from build123d import *

# Parameters (mm, degrees)
SKETCH1_R               = 60
BOSS_EXTRUDE1_DEPTH     = 1.5
SKETCH2_R               = 1.6
CUT_EXTRUDE1_DEPTH      = 2.5
MIRROR2_COPY_1_SKETCH_R = 1.6
MIRROR2_COPY_1_DEPTH    = 2.5
SKETCH3_W               = 3
SKETCH3_H               = 4
CUT_EXTRUDE2_DEPTH      = 4
LPATTERN1_COUNT         = 2
LPATTERN1_PITCH         = 8
MIRROR3_COPY_1_SKETCH_W = 3
MIRROR3_COPY_1_SKETCH_H = 4
MIRROR3_COPY_1_DEPTH    = 4
MIRROR4_COPY_1_SKETCH_W = 3
MIRROR4_COPY_1_SKETCH_H = 4
MIRROR4_COPY_1_DEPTH    = 4
MIRROR4_COPY_2_SKETCH_W = 3
MIRROR4_COPY_2_SKETCH_H = 4
MIRROR4_COPY_2_DEPTH    = 4
MIRROR4_COPY_3_SKETCH_W = 3
MIRROR4_COPY_3_SKETCH_H = 4
MIRROR4_COPY_3_DEPTH    = 4
CUT_EXTRUDE3_START      = -4
CUT_EXTRUDE3_DEPTH      = 5
CIRPATTERN1_COUNT       = 4


with BuildPart() as part:
    # Sketch1 → Boss-Extrude1 (new body, symmetric)
    with BuildSketch(Plane(origin=(0, 0, 0), x_dir=(1, 0, 0), z_dir=(0, 1, 0))):
        Circle(SKETCH1_R)
    extrude(amount=BOSS_EXTRUDE1_DEPTH, both=True)

    # Sketch2 → Cut-Extrude1 (cut, symmetric)
    with BuildSketch(Plane(origin=(0, 0, 0), x_dir=(1, 0, 0), z_dir=(0, 1, 0))):
        with Locations((54, 11)):
            Circle(SKETCH2_R)
    cut_extrude1 = extrude(amount=CUT_EXTRUDE1_DEPTH, both=True, mode=Mode.SUBTRACT)

    # Mirror1: Cut-Extrude1 across plane
    add(cut_extrude1.mirror(Plane(origin=(0, 0, 0), x_dir=(0, 0, 1), z_dir=(1, 0, 0))), mode=Mode.SUBTRACT)

    # Mirror2: Cut-Extrude1 across plane
    add(cut_extrude1.mirror(Plane.XY), mode=Mode.SUBTRACT)

    # Mirror2 copy 1 sketch → Mirror2 copy 1 (cut, symmetric)
    with BuildSketch(Plane(origin=(0, 0, 0), x_dir=(-1, 0, 0), z_dir=(0, 1, 0))):
        with Locations((54, 11)):
            Circle(MIRROR2_COPY_1_SKETCH_R)
    extrude(amount=MIRROR2_COPY_1_DEPTH, both=True, mode=Mode.SUBTRACT)

    # Sketch3 → Cut-Extrude2 (cut, through all)
    with BuildSketch(Plane(origin=(0, 1.5, 0), x_dir=(1, 0, 0), z_dir=(0, 1, 0))):
        with Locations((-8.5, 48)):
            Rectangle(SKETCH3_W, SKETCH3_H)
    cut_extrude2 = extrude(amount=-CUT_EXTRUDE2_DEPTH, mode=Mode.SUBTRACT)

    # LPattern1: Cut-Extrude2 ×2
    with Locations(*[(0, 0, i * LPATTERN1_PITCH) for i in range(1, LPATTERN1_COUNT)]):
        add(cut_extrude2, mode=Mode.SUBTRACT)

    # Mirror3: Cut-Extrude2 across plane
    add(cut_extrude2.mirror(Plane(origin=(0, 0, 0), x_dir=(0, 0, 1), z_dir=(1, 0, 0))), mode=Mode.SUBTRACT)

    # Mirror3 copy 1 sketch → Mirror3 copy 1 (cut, through all)
    with BuildSketch(Plane(origin=(0, 1.5, 8), x_dir=(-1, 0, 0), z_dir=(0, 1, 0))):
        with Locations((-8.5, -48)):
            Rectangle(MIRROR3_COPY_1_SKETCH_W, MIRROR3_COPY_1_SKETCH_H)
    extrude(amount=-MIRROR3_COPY_1_DEPTH, mode=Mode.SUBTRACT)

    # Mirror4: Cut-Extrude2 across plane
    add(cut_extrude2.mirror(Plane.XY), mode=Mode.SUBTRACT)

    # Mirror4 copy 1 sketch → Mirror4 copy 1 (cut, through all)
    with BuildSketch(Plane(origin=(0, 1.5, 0), x_dir=(-1, 0, 0), z_dir=(0, 1, 0))):
        with Locations((-8.5, 48)):
            Rectangle(MIRROR4_COPY_1_SKETCH_W, MIRROR4_COPY_1_SKETCH_H)
    extrude(amount=-MIRROR4_COPY_1_DEPTH, mode=Mode.SUBTRACT)

    # Mirror4 copy 2 sketch → Mirror4 copy 2 (cut, through all)
    with BuildSketch(Plane(origin=(0, 1.5, -8), x_dir=(-1, 0, 0), z_dir=(0, 1, 0))):
        with Locations((-8.5, 48)):
            Rectangle(MIRROR4_COPY_2_SKETCH_W, MIRROR4_COPY_2_SKETCH_H)
    extrude(amount=-MIRROR4_COPY_2_DEPTH, mode=Mode.SUBTRACT)

    # Mirror4 copy 3 sketch → Mirror4 copy 3 (cut, through all)
    with BuildSketch(Plane(origin=(0, 1.5, -8), x_dir=(1, 0, 0), z_dir=(0, 1, 0))):
        with Locations((-8.5, -48)):
            Rectangle(MIRROR4_COPY_3_SKETCH_W, MIRROR4_COPY_3_SKETCH_H)
    extrude(amount=-MIRROR4_COPY_3_DEPTH, mode=Mode.SUBTRACT)

    # Sketch4 → Cut-Extrude3 (cut)
    with BuildSketch(Plane(origin=(0, 1.5, 0), x_dir=(1, 0, 0), z_dir=(0, 1, 0)).offset(CUT_EXTRUDE3_START)):
        Polygon((27.223611076, 41.365746699), (41.365746699, 27.223611076), (43.487067043, 29.344931419), (29.344931419, 43.487067043), align=None)
    cut_extrude3 = extrude(amount=CUT_EXTRUDE3_DEPTH, mode=Mode.SUBTRACT)

    # CirPattern1: Cut-Extrude3 ×4 about axis
    cirpattern1_axis = Axis((0, 0, 0), (0, 1, 0))
    for i in range(1, CIRPATTERN1_COUNT):
        add(cut_extrude3.rotate(cirpattern1_axis, i * 360 / CIRPATTERN1_COUNT), mode=Mode.SUBTRACT)


solid = part.part
For this review, take the finished solid that the model builds, in its own axes (mm). Coordinates: 2 decimals unless noted, no trailing zeros. Loops run counter-clockwise (first coordinate to the right, second up) from the corner with the lowest first, then second, coordinate; pieces in that order, holes last. Notation, with made-up numbers: (15, 82) - (20, 82) arc R34 cw to (20, 121) - close; hole circle Ø3 at (34.5, -37). An arc over 180 degrees is marked (long way). Use a Markdown table: item, result. Add a question column.
Item 1: For line 1 (Z direction, x = 54, y = -0.7); line 2 (X direction, y = -0.3, z = -43); line 3 (Z direction, x = -36.5, y = -0.5), list the stretches that pass through material, from the lowest coordinate up.
Item 2: We need section D-D (x = 48.5). Give the boundary of the cut face in (y, z).
Item 3: We need section A-A (z = -11). Give the boundary of the cut face in (x, y).
Item 4: We need section C-C (y = -0.9). Give the number of separate pieces and of enclosed holes in the cut face, and give its area (3 significant figures).
Item 5: Insertion check: pin 1 Ø1.5 at (x, y) = (-8.5, -0.5) entering from +Z; pin 2 Ø0.9 at (y, z) = (0.5, 47.5) entering from -X; pin 3 Ø0.9 at (y, z) = (0.5, -39.5) entering from +X. Each pin has a flat end and moves straight along its axis. Give the tip position at first contact, or say it passes through.
Item 6: We need section B-B (x = 31). Give the boundary of the cut face in (y, z).
Results list:
| question | item | result |
|---|---|---|
| 1 | line 1 | z = -26.15 to -12.6, -9.4 to 9.4, 12.6 to 26.15 |
| 1 | line 2 | x = -41.84 to -29.83, -28.86 to 28.86, 29.83 to 41.84 |
| 1 | line 3 | z = -47.62 to -36.33, -32.09 to 32.09, 36.33 to 47.62 |
| 2 | outline | (-1.5, -35.32) - (1.5, -35.32) - (1.5, 35.32) - (-1.5, 35.32) - close |
| 3 | outline | (-58.98, -1.5) - (-55.6, -1.5) - (-55.6, 1.5) - (-58.98, 1.5) - close; (-52.4, -1.5) - (52.4, -1.5) - (52.4, 1.5) - (-52.4, 1.5) - close; (55.6, -1.5) - (58.98, -1.5) - (58.98, 1.5) - (55.6, 1.5) - close |
| 4 | separate pieces | 1 |
| 4 | enclosed holes | 16 |
| 4 | area | 10,900 mm^2 |
| 5 | pin 1 | stops at z = 59.5 |
| 5 | pin 2 | stops at x = -37.23 |
| 5 | pin 3 | stops at x = 45.55 |
| 6 | outline | (-1.5, -51.37) - (1.5, -51.37) - (1.5, -41.83) - (-1.5, -41.83) - close; (-1.5, -37.59) - (1.5, -37.59) - (1.5, 37.59) - (-1.5, 37.59) - close; (-1.5, 41.83) - (1.5, 41.83) - (1.5, 51.37) - (-1.5, 51.37) - close |
